```python
from build123d import *

# Parameters (mm, degrees)
BOSS_EXTRUDE1_DEPTH = 1.27
SKETCH2_W           = 6.604
SKETCH2_H           = 6.604
CUT_EXTRUDE1_DEPTH  = 37.010715072


with BuildPart() as part:
    # Sketch1 → Boss-Extrude1 (new, symmetric)
    with BuildSketch(Plane(origin=(0, 0, 0), x_dir=(1, 0, 0), z_dir=(0, 1, 0))):
        Polygon((0, -25.4), (0, 25.4), (-25.4, 25.4), (-25.4, 6.35), (-15.4, 6.35), (-15.4, -6.35), (-25.4, -6.35), (-25.4, -25.4), align=None)
    extrude(amount=BOSS_EXTRUDE1_DEPTH, both=True)

    # Sketch2 → Cut-Extrude1 (cut, through all)
    with BuildSketch(Plane(origin=(0, 1.27, 0), x_dir=(1, 0, 0), z_dir=(0, 1, 0))):
        with Locations((-3.302, 22.098)):
            Rectangle(SKETCH2_W, SKETCH2_H)
        with Locations((-16.002, 22.098)):
            Rectangle(SKETCH2_W, SKETCH2_H)
        with Locations((-16.002, -22.098)):
            Rectangle(SKETCH2_W, SKETCH2_H)
        with Locations((-3.302, -22.098)):
            Rectangle(SKETCH2_W, SKETCH2_H)
    extrude(amount=-CUT_EXTRUDE1_DEPTH, mode=Mode.SUBTRACT)


solid = part.part
```
Could you check a few things on this model? Use its own coordinates, in mm. A direction names the side the tool comes from. Coordinates: 2 decimals unless noted, no trailing zeros. Write each loop counter-clockwise with the first axis right and the second up, starting at its lowest first coordinate (ties: lowest second). Pieces come first, ordered by that corner, then holes. Notation, with made-up numbers: M 74.5,23.25 L 79.5,23.25 A23 cw 79.5,62.25 Z; hole C 8,32 d3. An arc over 180 degrees is marked long. Answer as CSV lines item,"result". Start each with the question number.
1) For P1, Ø1.5, axis at x = -4.5, y = 0.5, coming from the +Z side; P2, Ø0.8, axis at y = 0.5, z = 0.5, coming from the -X side; P3, Ø0.8, axis at y = 0, z = 23, coming from the +X side; P4, Ø1, axis at x = -13, y = 0, coming from the +Z side, each with a flat end and sliding along its axis, tell me the tip position at first contact or that it passes through.
2) I want a section at C-C, the plane y = 0.4. Please give me the cut outline in (x, z), and give its area (3 significant figures).
3) Please list where these lines run through material, in increasing order: line 1 (Z direction, x = -17, y = 1.1); line 2 (X direction, y = -0.1, z = 20); line 3 (Z direction, x = -6, y = 1.05). Write a range as from..to.
4) We'd pull the mould along X, two halves only. Please class faces 1 (the flat face through (-6.604, 0, 22)), 2 (the flat face through (-15.4, 0, 0)), 3 (the flat face through (-22, 0, 25.4)), 4 (the flat face through (-16, 0, 18.796)): +X half, -X half, draft (parallel to the pull), parting line (faces both ways), or undercut.
5) For faces 5 (the flat face through (-3, 0, 18.796)), 6 (the flat face through (-20, 0, -6.35)), 7 (the flat face through (-12.7, 0, 22)), 8 (the flat face through (-6.604, 0, -22)), 9 (the flat face through (-12.7, 0, -22)), which set-ups out of +Z, -Z, +X, -X, +Y, -Y let a thin tool reach every point of the face, with its end or its side?
6) I want a section at A-A, the plane x = -22.25. Please give me the cut outline in (y, z), and give its area (3 significant figures).
7) I want a section at B-B, the plane z = 20.5. Please give me the cut outline in (x, y).
8) I want a section at D-D, the plane x = -14. Please give me the cut outline in (y, z), and give its area (3 significant figures).
Data:
1,P1,"stops at z = 18.8"
1,P2,"stops at x = -15.4"
1,P3,"stops at x = -6.6"
1,P4,"stops at z = 25.4"
2,outline,"M -25.4,-25.4 L -19.3,-25.4 L -19.3,-18.8 L -12.7,-18.8 L -12.7,-25.4 L -6.6,-25.4 L -6.6,-18.8 L 0,-18.8 L 0,18.8 L -6.6,18.8 L -6.6,25.4 L -12.7,25.4 L -12.7,18.8 L -19.3,18.8 L -19.3,25.4 L -25.4,25.4 L -25.4,6.35 L -15.4,6.35 L -15.4,-6.35 L -25.4,-6.35 Z"
2,area,"989 mm^2"
3,line 1,"z = -18.8..-6.35, 6.35..18.8"
3,line 2,"x = -25.4..-19.3, -12.7..-6.6"
3,line 3,"z = -18.8..18.8"
4,face 1,"+X half"
4,face 2,"-X half"
4,face 3,"draft"
4,face 4,"undercut"
5,face 5,"+Z, +X, +Y, -Y"
5,face 6,"-X, +Y, -Y"
5,face 7,"+Z, +Y, -Y"
5,face 8,"-Z, +X, +Y, -Y"
5,face 9,"-Z, +Y, -Y"
6,outline,"M -1.27,-25.4 L 1.27,-25.4 L 1.27,-6.35 L -1.27,-6.35 Z; M -1.27,6.35 L 1.27,6.35 L 1.27,25.4 L -1.27,25.4 Z"
6,area,"96.8 mm^2"
7,outline,"M -25.4,-1.27 L -19.3,-1.27 L -19.3,1.27 L -25.4,1.27 Z; M -12.7,-1.27 L -6.6,-1.27 L -6.6,1.27 L -12.7,1.27 Z"
8,outline,"M -1.27,-18.8 L 1.27,-18.8 L 1.27,18.8 L -1.27,18.8 Z"
8,area,"95.5 mm^2"
